Design review of the part built by this model. Coordinates are the model's own, in mm. A direction names the side the tool comes from. Coordinates: 2 decimals unless noted, no trailing zeros. Loops run counter-clockwise (first coordinate to the right, second up) from the corner with the lowest first, then second, coordinate; pieces in that order, holes last. Notation, with made-up numbers: (50, 26.25) -> (87, 26.25) arc R34 cw to (87, 63.25) -> close; hole circle Ø9 at (66, -4). An arc over 180 degrees is marked (long way). One line per item, written item: value. Start each with the question number.
1. Machinability: for faces 1 (the flat face through (-35, -33, 4)), 2 (the flat face through (39.396, 22.179, 4.437)), 3 (the flat face through (10.674, 46.577, 4.437)), which of the approach directions +Z, -Z, +X, -X, +Y, -Y give a long, thin tool a straight path to every point of the face, cutting with its end or side? Answer none if there is none.
2. Insertion check: pin 1 (4.5 mm diameter, centred on y = -39, z = 4.5, fed in from -X); pin 2 (4 mm diameter, centred on x = 35.5, y = 21, fed in from -Z); pin 3 (3 mm diameter, centred on y = -26.5, z = 7.5, fed in from +X); pin 4 (9.5 mm diameter, centred on x = 0, y = 0, fed in from -Z). Each pin has a flat end and moves straight along its axis. Give the tip position at first contact, or say it passes through.
3. Draft analysis for pull direction Y (two halves, no side actions). For faces 4 (the cylindrical face through (-1.73, -7.81, 4.56)), 5 (the flat face through (-10.674, 46.577, 4.437)), 6 (the flat face through (35, -33, 4)), 7 (the flat face through (0, -45.207, 4)), state which applies: pulls with the +Y half, pulls with the -Y half, needs draft (parallel to the pull), parting line crosses it, or undercut.
4. For probe 1 along Y at (x, z) = (0, 3); probe 2 along X at (y, z) = (-21.5, 6.25); probe 3 along X at (y, z) = (-6.5, 8.75), list the stretches that pass through material, from the lowest coordinate up.
5. Add section D-D on x = -30.5. Write out the cut boundary in (y, z), plus the area to 3 significant figures.
6. Add section B-B on y = 43.5. Write out the cut boundary in (x, z).
7. Add section A-A on z = 2.25. Write out the cut boundary in (x, y), plus the area to 3 significant figures.
8. Add section C-C on y = 0. Write out the cut boundary in (x, z).
```python
from build123d import *

# Parameters (mm, degrees)
F1_DEPTH = 9
F2_DEPTH = 25
F3_DEPTH = 25
F4_DEPTH = 25
F5_R     = 8
F6_DEPTH = 25


with BuildPart() as f1:
    # F0 (on Top) → F1 (new body)
    with BuildSketch(Plane.XY):
        Polygon((-35, -20.2072594216), (35, -20.2072594216), (0, 40.4145188433), align=None)
    extrude(amount=F1_DEPTH)

    # F2 (add): a face of the model
    f2_faces = [f1.faces().sort_by_distance(p)[0] for p in [
        (0, -20.2072594216, 4.5),
    ]]
    extrude(f2_faces, amount=F2_DEPTH)

    # F3 (add): a face of the model
    f3_faces = [f1.faces().sort_by_distance(p)[0] for p in [
        (17.5, 10.1036297108, 4.5),
    ]]
    extrude(f3_faces, amount=F3_DEPTH)

    # F4 (add): a face of the model
    f4_faces = [f1.faces().sort_by_distance(p)[0] for p in [
        (-17.5, 10.1036297108, 4.5),
    ]]
    extrude(f4_faces, amount=F4_DEPTH)

    # F5 (on face) → F6 (cut)
    with BuildSketch(Plane.XY.offset(9)):
        Circle(F5_R)
    extrude(amount=-F6_DEPTH, mode=Mode.SUBTRACT)


solid = f1.part
```
Worked answers:
1. face 1: +Z, -Z, -X, -Y
1. face 2: +Z, -Z, +X, +Y
1. face 3: +Z, -Z, +Y
2. pin 1: stops at x = -35
2. pin 2: stops at z = 0
2. pin 3: stops at x = 35
2. pin 4: passes through
3. face 4: undercut
3. face 5: pulls with the +Y half
3. face 6: needs draft
3. face 7: pulls with the -Y half
4. probe 1: y = -45.21 to -8, 8 to 40.41
4. probe 2: x = -35 to 35
4. probe 3: x = -55.95 to -4.66, 4.66 to 55.95
5. outline: (-45.21, 0) -> (37.59, 0) -> (37.59, 9) -> (-45.21, 9) -> close
5. area: 745 mm²
6. outline: (-27.09, 0) -> (-5.34, 0) -> (-5.34, 9) -> (-27.09, 9) -> close; (5.34, 0) -> (27.09, 0) -> (27.09, 9) -> (5.34, 9) -> close
7. outline: (-56.65, -7.71) -> (-35, -20.21) -> (-35, -45.21) -> (35, -45.21) -> (35, -20.21) -> (56.65, -7.71) -> (21.65, 52.91) -> (0, 40.41) -> (-21.65, 52.91) -> close; hole circle Ø16 at (0, 0)
7. area: 7,170 mm²
8. outline: (-52.2, 0) -> (-8, 0) -> (-8, 9) -> (-52.2, 9) -> close; (8, 0) -> (52.2, 0) -> (52.2, 9) -> (8, 9) -> close
